from build123d import *

# Parameters (mm, degrees)
SKETCH1_W           = 6
SKETCH1_H           = 5
BOSS_EXTRUDE1_DEPTH = 3.5
SKETCH1_3_W         = 3.75
SKETCH1_3_H         = 5
BOSS_EXTRUDE2_DEPTH = 1
CUT_EXTRUDE1_START  = -2.5
SKETCH2_W           = 2.1
SKETCH2_H           = 3
CUT_EXTRUDE1_DEPTH  = 2.5
SKETCH3_W           = 0.441524735
SKETCH3_H           = 5
SKETCH3_W_2         = 0.441524734
CUT_EXTRUDE2_DEPTH  = 0.2


with BuildPart() as part:
    # Sketch1 → Boss-Extrude1 (new body)
    with BuildSketch(Plane.XY):
        Rectangle(SKETCH1_W, SKETCH1_H)
    extrude(amount=BOSS_EXTRUDE1_DEPTH)

    # Sketch1<3> → Boss-Extrude2 (add)
    with BuildSketch(Plane.XY):
        with Locations((-4.875, 0)):
            Rectangle(SKETCH1_3_W, SKETCH1_3_H)
        with Locations((4.875, 0)):
            Rectangle(SKETCH1_3_W, SKETCH1_3_H)
    extrude(amount=BOSS_EXTRUDE2_DEPTH)

    # Sketch2 → Cut-Extrude1 (cut)
    with BuildSketch(Plane(origin=(0, 0, 0), x_dir=(-1, 0, 0), z_dir=(0, 0, -1)).offset(CUT_EXTRUDE1_START)):
        Rectangle(SKETCH2_W, SKETCH2_H)
    extrude(amount=CUT_EXTRUDE1_DEPTH, mode=Mode.SUBTRACT)

    # Sketch3 → Cut-Extrude2 (cut)
    with BuildSketch(Plane.XY.offset(3.5)):
        with Locations((-2.64914841, 0)):
            Rectangle(SKETCH3_W, SKETCH3_H)
        with Locations((-1.766098939, 0)):
            Rectangle(SKETCH3_W, SKETCH3_H)
        with Locations((-0.88304947, 0)):
            Rectangle(SKETCH3_W, SKETCH3_H)
        Rectangle(SKETCH3_W_2, SKETCH3_H)
        with Locations((0.88304947, 0)):
            Rectangle(SKETCH3_W, SKETCH3_H)
        with Locations((1.766098939, 0)):
            Rectangle(SKETCH3_W, SKETCH3_H)
        with Locations((2.64914841, 0)):
            Rectangle(SKETCH3_W, SKETCH3_H)
    extrude(amount=-CUT_EXTRUDE2_DEPTH, mode=Mode.SUBTRACT)


solid = part.part
Could you check a few things on this model? Use its own coordinates, in mm. A direction names the side the tool comes from. Coordinates: 2 decimals unless noted, no trailing zeros. Loops run counter-clockwise (first coordinate to the right, second up) from the corner with the lowest first, then second, coordinate; pieces in that order, holes last.
1. Imagine slicing it at D-D (z = 0.7). Please give me the cut outline in (x, y), and give its area (3 significant figures).
2. I need wall thicknesses on L1, parallel to X at y = 0.65, z = 1.45; L2, parallel to X at y = -1.1, z = 0.5; L3, parallel to Z at x = -4.25, y = 1.75. Which ranges of each line are inside material? Lowest first, please.
3. Imagine slicing it at B-B (x = 0.5). Please give me the cut outline in (y, z), and give its area (4 significant figures).
4. Imagine slicing it at C-C (z = 3.05). Please give me the cut outline in (x, y), and give its area (3 significant figures).
5. We'd pull the mould along Y, two halves only. Please class faces 1 (the face through (0, 2.5, 1)), 2 (the face through (0, 1.5, 1)), 3 (the face through (3, 0, 2)): released by +Y, released by -Y, zero draft, split by the parting line, or undercut.
6. For P1, Ø2, axis at y = 1, z = 2.5, coming from the -X side; P2, Ø0.6, axis at x = -0.5, y = 0, coming from the -Z side, each with a flat end and sliding along its axis, tell me the tip position at first contact or that it passes through.
7. For faces 4 (the face through (-3, 0, 2)), 5 (the face through (-2, 0, 0)), 6 (the face through (5, 0, 1)), 7 (the face through (-1.05, 0, 1)), which set-ups out of +Z, -Z, +X, -X, +Y, -Y let a thin tool reach every point of the face, with its end or its side?
8. Imagine slicing it at A-A (z = 1.5). Please give me the cut outline in (x, y).
Computed values:
1. outline: (-6.75, -2.5) - (6.75, -2.5) - (6.75, 2.5) - (-6.75, 2.5) - close; hole (-1.05, -1.5) - (1.05, -1.5) - (1.05, 1.5) - (-1.05, 1.5) - close
1. area: 61.2 mm2
2. L1: x = -3 to -1.05, 1.05 to 3
2. L2: x = -6.75 to -1.05, 1.05 to 6.75
2. L3: z = 0 to 1
3. outline: (-2.5, 0) - (-1.5, 0) - (-1.5, 2.5) - (1.5, 2.5) - (1.5, 0) - (2.5, 0) - (2.5, 3.5) - (-2.5, 3.5) - close
3. area: 10.00 mm2
4. outline: (-3, -2.5) - (3, -2.5) - (3, 2.5) - (-3, 2.5) - close
4. area: 30.0 mm2
5. face 1: released by +Y
5. face 2: undercut
5. face 3: zero draft
6. P1: stops at x = -3
6. P2: stops at z = 2.5
7. face 4: +Z, -X, +Y, -Y
7. face 5: -Z, +X, -X, +Y, -Y
7. face 6: +Z, +X, +Y, -Y
7. face 7: -Z
8. outline: (-3, -2.5) - (3, -2.5) - (3, 2.5) - (-3, 2.5) - close; hole (-1.05, -1.5) - (1.05, -1.5) - (1.05, 1.5) - (-1.05, 1.5) - close
